The model under review builds one solid part; all positions refer to its coordinate system, in mm. A direction names the side the tool comes from. Coordinates: 2 decimals unless noted, no trailing zeros. Loops run counter-clockwise (first coordinate to the right, second up) from the corner with the lowest first, then second, coordinate; pieces in that order, holes last. Notation, with made-up numbers: M 65,-32.75 L 90,-32.75 A22 cw 90,-22.75 Z; hole C 27.5,51.5 d3. An arc over 180 degrees is marked long. One line per item, written item: value.
```python
from build123d import *

# Parameters (mm, degrees)
SKETCH_1_R          = 1.1
EXTRUDE_1_DEPTH     = 6
EXTRUDE_2_DEPTH     = 2.5
SKETCH_2_R          = 2.1
CUT_EXTRUDE_1_DEPTH = 2.8
CHAMFER_1_SIZE      = 5
CHAMFER_2_SIZE      = 5
CHAMFER_2_SIZE_2    = 20.362059886


with BuildPart() as part:
    # 스케치1 → 보스-돌출1 (new body)
    # profile 1 of 3: a face of its own
    with BuildSketch(Plane.XY):
        with BuildLine():
            Line((81.914344353, -51.358871931), (21.75, -9.23))
            Line((21.75, -9.23), (5.029063305, -9.23))
            Line((5.029063305, -9.23), (14.961256377, -16.641470968))
            ThreePointArc((14.961256377, -16.641470968), (0, -21.138080256), (-14.961256377, -16.641470968))
            Line((-14.961256377, -16.641470968), (-5.029063305, -9.23))
            Line((-5.029063305, -9.23), (-21.75, -9.23))
            Line((-21.75, -9.23), (-81.914344353, -51.358871931))
            ThreePointArc((-81.914344353, -51.358871931), (0, -94), (81.914344353, -51.358871931))
        make_face()
        with BuildLine():
            ThreePointArc((-23.561943602, -22.706651125), (-22.285743682, -23.708292339), (-20.967016307, -24.653241791))
            Line((-20.967016307, -24.653241791), (-44.754559097, -72.083477382))
            ThreePointArc((-44.754559097, -72.083477382), (-56.906680731, -63.725387688), (-67.530529729, -53.494769135))
            Line((-67.530529729, -53.494769135), (-23.561943602, -22.706651125))
        make_face(mode=Mode.SUBTRACT)
        with BuildLine():
            ThreePointArc((-12.028210812, -29.136293911), (-8.554644148, -30.139383899), (-5, -30.799959309))
            Line((-5, -30.799959309), (-5, -83.861003778))
            ThreePointArc((-5, -83.861003778), (-20.731227032, -81.579770642), (-35.815753602, -76.566529502))
            Line((-35.815753602, -76.566529502), (-12.028210812, -29.136293911))
        make_face(mode=Mode.SUBTRACT)
        with BuildLine():
            Line((5, -83.861003778), (5, -30.799959309))
            ThreePointArc((5, -30.799959309), (9.099152416, -30.006144343), (13.08329394, -28.757221189))
            Line((13.08329394, -28.757221189), (38.291645519, -75.447835351))
            ThreePointArc((38.291645519, -75.447835351), (22.050782156, -81.256879421), (5, -83.861003778))
        make_face(mode=Mode.SUBTRACT)
        with BuildLine():
            ThreePointArc((21.88270877, -24.006400351), (22.731617723, -23.36853011), (23.561943602, -22.706651125))
            Line((23.561943602, -22.706651125), (67.530529729, -53.494769135))
            ThreePointArc((67.530529729, -53.494769135), (57.952623233, -62.858503182), (47.09106035, -70.697014513))
            Line((47.09106035, -70.697014513), (21.88270877, -24.006400351))
        make_face(mode=Mode.SUBTRACT)
    # profile 2 of 3: a face of its own
    with BuildSketch(Plane.XY):
        Polygon((5.029063305, -9.23), (21.75, -9.23), (0, 6), (-21.75, -9.23), (-5.029063305, -9.23), align=None)
        with Locations((-5.1, 0)):
            Circle(SKETCH_1_R, mode=Mode.SUBTRACT)
        with Locations((5.1, 0)):
            Circle(SKETCH_1_R, mode=Mode.SUBTRACT)
    # profile 3 of 3: a face of its own
    with BuildSketch(Plane.XY):
        Polygon((21.75, -9.23), (21.75, 21.23), (-21.75, 21.23), (-21.75, -9.23), (0, 6), align=None)
        with Locations((-15.1, 0)):
            Circle(SKETCH_1_R, mode=Mode.SUBTRACT)
        with Locations((-15.1, 12)):
            Circle(SKETCH_1_R, mode=Mode.SUBTRACT)
        with Locations((-5.1, 12)):
            Circle(SKETCH_1_R, mode=Mode.SUBTRACT)
        with Locations((15.1, 0)):
            Circle(SKETCH_1_R, mode=Mode.SUBTRACT)
        with Locations((5.1, 12)):
            Circle(SKETCH_1_R, mode=Mode.SUBTRACT)
        with Locations((15.1, 12)):
            Circle(SKETCH_1_R, mode=Mode.SUBTRACT)
    extrude(amount=EXTRUDE_1_DEPTH)

    # 스케치1<3> → 보스-돌출2 (add)
    with BuildSketch(Plane.XY):
        with BuildLine():
            Line((-23.561943602, -22.706651125), (-67.530529729, -53.494769135))
            ThreePointArc((-67.530529729, -53.494769135), (-56.906680731, -63.725387688), (-44.754559097, -72.083477382))
            Line((-44.754559097, -72.083477382), (-20.967016307, -24.653241791))
            ThreePointArc((-20.967016307, -24.653241791), (-22.285743682, -23.708292339), (-23.561943602, -22.706651125))
        make_face()
        with BuildLine():
            ThreePointArc((-12.028210812, -29.136293911), (-8.554644148, -30.139383899), (-5, -30.799959309))
            Line((-5, -30.799959309), (-5, -83.861003778))
            ThreePointArc((-5, -83.861003778), (-20.731227032, -81.579770642), (-35.815753602, -76.566529502))
            Line((-35.815753602, -76.566529502), (-12.028210812, -29.136293911))
        make_face()
        with BuildLine():
            ThreePointArc((5, -30.799959309), (9.099152416, -30.006144343), (13.08329394, -28.757221189))
            Line((13.08329394, -28.757221189), (38.291645519, -75.447835351))
            ThreePointArc((38.291645519, -75.447835351), (22.050782156, -81.256879421), (5, -83.861003778))
            Line((5, -83.861003778), (5, -30.799959309))
        make_face()
        with BuildLine():
            ThreePointArc((21.88270877, -24.006400351), (22.731617723, -23.36853011), (23.561943602, -22.706651125))
            Line((23.561943602, -22.706651125), (67.530529729, -53.494769135))
            ThreePointArc((67.530529729, -53.494769135), (57.952623233, -62.858503182), (47.09106035, -70.697014513))
            Line((47.09106035, -70.697014513), (21.88270877, -24.006400351))
        make_face()
        with BuildLine():
            Line((14.961256377, -16.641470968), (5.029063305, -9.23))
            Line((5.029063305, -9.23), (-5.029063305, -9.23))
            Line((-5.029063305, -9.23), (-14.961256377, -16.641470968))
            ThreePointArc((-14.961256377, -16.641470968), (0, -21.138080256), (14.961256377, -16.641470968))
        make_face()
    extrude(amount=EXTRUDE_2_DEPTH)

    # 스케치2 → 컷-돌출1 (cut)
    with BuildSketch(Plane.XY.offset(6)):
        with Locations((-15.1, 12)):
            Circle(SKETCH_2_R)
        with Locations((-5.1, 12)):
            Circle(SKETCH_2_R)
        with Locations((5.1, 12)):
            Circle(SKETCH_2_R)
        with Locations((15.1, 12)):
            Circle(SKETCH_2_R)
        with Locations((15.1, 0)):
            Circle(SKETCH_2_R)
        with Locations((5.1, 0)):
            Circle(SKETCH_2_R)
        with Locations((-5.1, 0)):
            Circle(SKETCH_2_R)
        with Locations((-15.1, 0)):
            Circle(SKETCH_2_R)
    extrude(amount=-CUT_EXTRUDE_1_DEPTH, mode=Mode.SUBTRACT)

    # 모따기1
    chamfer_1_edges = [part.edges().sort_by_distance(p)[0] for p in [
        (-21.75, 21.23, 3),
        (21.75, 21.23, 3),
    ]]
    chamfer(chamfer_1_edges, length=CHAMFER_1_SIZE)

    # 모따기2
    # the kernel refuses this chamfer: 20.362059886, 5 mm, written as the material it adds along each edge
    with BuildSketch(Plane(origin=(-21.75, -9.23, 0), x_dir=(-0.8191434435315306, -0.573588719309669, 0), z_dir=(0, 0, 1))) as chamfer_2_piece_1:
        Polygon((CHAMFER_2_SIZE, 0), (-CHAMFER_2_SIZE_2 * 0.573588719322, -CHAMFER_2_SIZE_2 * 0.819143443549), (0, 0), align=None)
    extrude(amount=6)
    with BuildSketch(Plane(origin=(21.75, -9.23, 0), x_dir=(0, 1, 0), z_dir=(0, 0, 1))) as chamfer_2_piece_2:
        Polygon((CHAMFER_2_SIZE_2, 0), (-CHAMFER_2_SIZE * 0.57358871931, -CHAMFER_2_SIZE * 0.819143443532), (0, 0), align=None)
    extrude(amount=6)
    # the kernel refuses this chamfer: 20.362059886, 5 mm, written as the material it takes off along each edge
    with BuildSketch(Plane(origin=(81.914344353, -51.358871931, -12.85841494), x_dir=(-0.8191434435315298, 0.5735887193096699, 0), z_dir=(0, 0, 1))) as chamfer_2_2_piece_1:
        with BuildLine():
            Line((CHAMFER_2_SIZE, 0), (0.119182901, 4.880817099))
            ThreePointArc((0.119182901, 4.880817099), (0.031506692, 2.510048959), (0, 0))
            Line((0, 0), (CHAMFER_2_SIZE, 0))
        make_face()
    extrude(amount=31.71682988, mode=Mode.SUBTRACT)
    with BuildSketch(Plane(origin=(-81.914344353, -51.358871931, -12.85841494), x_dir=(0.5934141945147567, -0.8048972566411209, 0), z_dir=(0, 0, 1))) as chamfer_2_2_piece_2:
        with BuildLine():
            Line((4.882272025, 0), (CHAMFER_2_SIZE * 0.0244113601227, CHAMFER_2_SIZE * 0.999701998346))
            Line((CHAMFER_2_SIZE * 0.0244113601227, CHAMFER_2_SIZE * 0.999701998346), (0, 0))
            ThreePointArc((0, 0), (2.510070082, -0.029776406), (4.882272025, 0))
        make_face()
    extrude(amount=31.71682988, mode=Mode.SUBTRACT)


solid = part.part
```
(1) Add section C-C on y = -45. State the section outline as (x, z) points.
Checks:
outline: M -72.83,0 L 72.83,0 L 72.83,6 L 55.4,6 L 55.4,2.5 L 33.22,2.5 L 33.22,6 L 21.85,6 L 21.85,2.5 L 5,2.5 L 5,6 L -5,6 L -5,2.5 L -19.98,2.5 L -19.98,6 L -31.17,6 L -31.17,2.5 L -55.4,2.5 L -55.4,6 L -72.83,6 Z
(2) Insertion check: pin 1 Ø5 at (x, y) = (15.1, 12) entering from -Z; pin 2 Ø3 at (x, z) = (3, 4) entering from -Y; pin 3 Ø3 at (x, z) = (61, 2) entering from +Y; pin 4 Ø1.5 at (y, z) = (-71, 1) entering from +X. Each pin has a flat end and moves straight along its axis. Give the tip position at first contact, or say it passes through.
Checks:
pin 1: z = 0
pin 2: y = -93.99
pin 3: y = -35.66
pin 4: x = 64.7
(3) To check wall thickness, follow L1, parallel to X at y = -60, z = 3.25; L2, parallel to Y at x = -5.1, z = 2.3; L3, parallel to Y at x = -5.1, z = 5.3. State the ranges of each line that lie inside material, in increasing order. Write a range as [from, to].
Checks:
L1: [-75.13, -61.19], [-38.69, -27.51], [-5, 5], [29.95, 41.32], [61.19, 75.13]
L2: [-93.87, -1.1], [1.1, 10.9], [13.1, 21.23]
L3: [-93.87, -83.86], [-30.79, -20.65], [-9.28, -2.1], [2.1, 9.9], [14.1, 21.23]
(4) Draft analysis for pull direction Y (two halves, no side actions). For faces 1 (the face through (-1, -36, 6)), 2 (the face through (58.096, -62.737, 4.226)), 3 (the face through (-23.827, -0.646, 2.958)), state which applies: pulls with the +Y half, pulls with the -Y half, needs draft (parallel to the pull), parting line crosses it, or undercut.
Checks:
face 1: needs draft
face 2: undercut
face 3: pulls with the +Y half
(5) Tool access review of faces 4 (the face through (-19.28, 18.7, 2.96)), 5 (the face through (-45, -47, 2.5)): name each direction out of +Z, -Z, +X, -X, +Y, -Y from which nothing blocks a thin tool from reaching the whole face with its end or side.
Checks:
face 4: +Z, -Z, -X, +Y
face 5: +Z
(6) Add section B-B on y = -60. State the section outline as (x, z) points, then the cut area to 3 significant figures.
Checks:
outline: M -75.13,0 L 75.13,0 L 75.13,6 L 61.19,6 L 61.19,2.5 L 41.32,2.5 L 41.32,6 L 29.95,6 L 29.95,2.5 L 5,2.5 L 5,6 L -5,6 L -5,2.5 L -27.51,2.5 L -27.51,6 L -38.69,6 L -38.69,2.5 L -61.19,2.5 L -61.19,6 L -75.13,6 Z
area: 587 mm^2
(7) Add section A-A on z = 4.75. State how many separate pieces and enclosed holes the cut face has, then the cut area to 3 significant figures.
Checks:
separate pieces: 1
enclosed holes: 13
area: 6,480 mm^2
